Part model, mm, in its own coordinate system. A direction names the side the tool comes from. Coordinates: 2 decimals unless noted, no trailing zeros. Loops run counter-clockwise (first coordinate to the right, second up) from the corner with the lowest first, then second, coordinate; pieces in that order, holes last. Notation, with made-up numbers: M -30.75,28.25 L 15.25,28.25 A34 ccw 15.25,66.25 Z; hole C -28,8 d6. An arc over 180 degrees is marked long. Use a Markdown table: item, result. Add a question column.
1) Band-saw the part on C-C (z = 120). List the corners of the cut face in (x, y), plus the area to 3 significant figures.
2) Tool access for faces 1 (the flat face through (0, 17.5, 195)), 2 (the flat face through (0, -14.5, 195)): list every direction of +Z, -Z, +X, -X, +Y, -Y with a clear straight run to the whole face (end or side of a thin tool).
3) Band-saw the part on B-B (y = -8). List the corners of the cut face in (x, z).
4) Wall check: probe 1 along Y at (x, z) = (3.5, 145); probe 2 along X at (y, z) = (-14, 293). Give the ranges that are in metal, low to high. Write a range as from..to.
5) Band-saw the part on A-A (x = -5). List the corners of the cut face in (y, z).
6) Pin check, flat tips, straight feed: pin 1 Ø6 at (x, y) = (6, 13.5) entering from +Z; pin 2 Ø8 at (x, y) = (12, -10) entering from +Z. Stop position of each tip, or through.
7) Pull direction Y, two halves, no side cores. Call faces 3 (the flat face through (0, -17.5, 195)), 4 (the flat face through (-14.5, 0, 195)), 5 (the flat face through (14.5, 0, 195)), 6 (the flat face through (0, 15, 395)): released by +Y, released by -Y, zero draft, split by the parting line, or undercut.
Autodesk Inventor part; units mm, degrees
ref_plane "Start plane" through (0, 0, -17.5) normal (0, 0, 1) x (1, 0, 0)
ref_plane "End plane" through (0, 0, 412.5) normal (0, 0, 1) x (1, 0, 0)
ref_plane "Work Plane12" through (0, 180, -17.5) normal (0, 0, -1) x (-1, 0, 0)
ref_plane "Start plane" through (0, 0, -17.5) normal (0, 0, 1) x (1, 0, 0)
ref_plane "End plane" through (0, 0, 412.5) normal (0, 0, 1) x (1, 0, 0)
sketch "Sketch" plane through (0, 0, 0) normal (0, 0, 1) x (1, 0, 0)
  line L0 (-17.5, -11.5) -> (-17.5, 11.5)
  line L1 (-11.5, 17.5) -> (11.5, 17.5)
  line L2 (17.5, 11.5) -> (17.5, -11.5)
  line L3 (11.5, -17.5) -> (-11.5, -17.5)
  arc A0 (-17.5, -11.5) -> (-11.5, -17.5) centre (-11.5, -11.5) ccw
  arc A1 (-11.5, 17.5) -> (-17.5, 11.5) centre (-11.5, 11.5) ccw
  arc A2 (17.5, 11.5) -> (11.5, 17.5) centre (11.5, 11.5) ccw
  arc A3 (11.5, -17.5) -> (17.5, -11.5) centre (11.5, -11.5) ccw
  arc A4 (-11.5, 14.5) -> (-14.5, 11.5) centre (-11.5, 11.5) ccw
  line L4 (-11.5, 14.5) -> (11.5, 14.5)
  arc A5 (14.5, 11.5) -> (11.5, 14.5) centre (11.5, 11.5) ccw
  line L5 (14.5, 11.5) -> (14.5, -11.5)
  arc A6 (11.5, -14.5) -> (14.5, -11.5) centre (11.5, -11.5) ccw
  line L6 (11.5, -14.5) -> (-11.5, -14.5)
  arc A7 (-14.5, -11.5) -> (-11.5, -14.5) centre (-11.5, -11.5) ccw
  line L7 (-14.5, -11.5) -> (-14.5, 11.5)
  line L8 (0, 25.6598) -> (0, -25.6598) construction
  line L9 (-25.6598, 0) -> (25.6598, 0) construction
  dimension "d7" = 6
  dimension "d10" = 35
  dimension "d11" = 35
  dimension "d12" = 3
  dimension "d15" = 17.5
  dimension "d16" = 17.5
extrude "Body" add sketch "Sketch" along normal up to surface (430 mm away) from surface at -17.5
sketch "Sketch3" plane through (0, 0, 0) normal (0, 0, 1) x (1, 0, 0)
  line L0 (0, 0) -> (10, 0)
ref_plane "Work Plane3" through (0, 0, 0) normal (0, -1, 0) x (1, 0, 0)
sketch "Sketch4" plane through (0, 0, 0) normal (0, -1, 0) x (1, 0, 0)
  line L0 (-2, -17.5) -> (12, -17.5)
  line L1 (-2, 412.5) -> (12, 412.5)
  dimension "d18" = 430
ref_plane "Work Plane12" through (0, 180, -17.5) normal (0, 0, -1) x (-1, 0, 0)
split "Split6" plane through (0, 180, -17.5) removes the side toward (0, 0, -1)
ref_plane "Work Plane13" through (17.5, 0, -17.5) normal (-0.7071, 0, -0.7071) x (-0.7071, 0, 0.7071)
split "Split7" plane through (17.5, 0, -17.5) removes the side toward (-0.7071, 0, -0.7071)
ref_plane "Work Plane14" through (17.5, 0, 412.5) normal (-0.7071, 0, 0.7071) x (0.7071, 0, 0.7071)
split "Split8" plane through (17.5, 0, 412.5) removes the side toward (-0.7071, 0, 0.7071)
equation "\"d7\" = G_IR"
equation "\"d10\" = G_H"
equation "\"d11\" = G_W"
equation "\"d12\" = G_T"
equation "\"d15\" = 0.5 * d10"
equation "\"d16\" = 0.5 * d11"
equation "\"d3\" = G_L"
equation "\"G_W\" = 35"
equation "\"G_H\" = 35"
equation "\"G_T\" = 3"
equation "\"G_IR\" = 6"
equation "\"G_L\" = d18"
equation "\"G_OFFSET_START\" = 17.5"
equation "\"G_OFFSET_END\" = 17.5"
equation "\"d13\" = -G_OFFSET_START"
equation "\"d14\" = G_OFFSET_END + B_L"
equation "\"B_L\" = 395"
properties part number "AS 1163 - C350L0 35x35x3.0 SHS - 430" material "Steel, Mild"
Entries:
| question | item | result |
|---|---|---|
| 1 | outline | M -17.5,-11.5 A6 ccw -11.5,-17.5 L 11.5,-17.5 A6 ccw 17.5,-11.5 L 17.5,11.5 A6 ccw 11.5,17.5 L -11.5,17.5 A6 ccw -17.5,11.5 Z; hole M -14.5,-11.5 A3 ccw -11.5,-14.5 L 11.5,-14.5 A3 ccw 14.5,-11.5 L 14.5,11.5 A3 ccw 11.5,14.5 L -11.5,14.5 A3 ccw -14.5,11.5 Z |
| 1 | area | 361 mm2 |
| 2 | face 1 | +Z, -Z, +X, -X, +Y |
| 2 | face 2 | +Z, -Z |
| 3 | outline | M -17.5,17.5 L -14.5,14.5 L -14.5,380.5 L -17.5,377.5 Z; M 14.5,-14.5 L 17.5,-17.5 L 17.5,412.5 L 14.5,409.5 Z |
| 4 | probe 1 | -17.5..-14.5, 14.5..17.5 |
| 4 | probe 2 | -16.95..-13.16, 13.16..16.95 |
| 5 | outline | M -17.5,5 L -14.5,5 L -14.5,390 L -17.5,390 Z; M 14.5,5 L 17.5,5 L 17.5,390 L 14.5,390 Z |
| 6 | pin 1 | z = 403.83 |
| 6 | pin 2 | z = 411 |
| 7 | face 3 | released by -Y |
| 7 | face 4 | undercut |
| 7 | face 5 | undercut |
| 7 | face 6 | zero draft |
